Autodesk Inventor part; units mm, degrees
ref_plane "YZ Plane" through (0, 0, 0) normal (1, 0, 0) x (0, 1, 0)
ref_plane "XZ Plane" through (0, 0, 0) normal (0, 1, 0) x (-1, 0, 0)
ref_plane "XY Plane" through (0, 0, 0) normal (0, 0, 1) x (1, 0, 0)
sketch "草图1" plane through (0, 0, 0) normal (0, 0, 1) x (1, 0, 0)
  circle A0 centre (0, 0) radius 45
  dimension "d0" = 90
extrude "拉伸1" add sketch "草图1" along normal blind 7
sketch "草图2" plane through (0, 0, 7) normal (0, 0, 1) x (1, 0, 0)
  circle A0 centre (0, 0) radius 26
  circle A1 centre (0, 0) radius 21
  dimension "d3" = 52
  dimension "d4" = 42
extrude "拉伸2" add sketch "草图2" along normal blind 8
sketch "草图3" plane through (0, 0, 15) normal (0, 0, 1) x (1, 0, 0)
  circle A0 centre (0, 0) radius 26
  circle A1 centre (0, 0) radius 25
  dimension "d7" = 52
  dimension "d8" = 50
extrude "拉伸3" cut sketch "草图3" against normal blind 2
sketch "草图4" plane through (0, 0, 7) normal (0, 0, 1) x (1, 0, 0)
  circle A0 centre (0, 0) radius 13
  dimension "d11" = 26
extrude "拉伸4" cut sketch "草图4" against normal through all
sketch "草图5" plane through (0, 0, 0) normal (0, 0, -1) x (-1, 0, 0)
  circle A0 centre (0, -35.5) radius 2.5
  circle A1 centre (35.5, 0) radius 2.5
  circle A2 centre (-35.5, 0) radius 2.5
  circle A3 centre (0, 35.5) radius 2.5
  line L0 (0, 0) -> (-3.8614, 0)
  line L1 (0, 0) -> (0, -7.2667)
  dimension "d15" = 5
  dimension "d16" = 5
  dimension "d17" = 5
  dimension "d18" = 5
  dimension "d19" = 35.5
  dimension "d20" = 35.5
  dimension "d21" = 35.5
  dimension "d22" = 35.5
  dimension "d23" = 7.2667
  dimension "d24" = 3.8614
extrude "拉伸5" cut sketch "草图5" against normal through all
sketch "草图6" plane through (0, 0, 0) normal (0, 0, -1) x (-1, 0, 0)
  circle A0 centre (0, 0) radius 22.5
  dimension "d27" = 45
extrude "拉伸6" cut sketch "草图6" against normal blind 1
fillet "圆角1" radius 0.5 2 edges at (22.5, 0, 0) (22.5, 0, 1)
equation "\"d12\" = d11"
properties part number "装填盘轴盖"
Geometry: final body of the model. Coordinates: model frame, mm. A direction names the side the tool comes from. Coordinates: 2 decimals unless noted, no trailing zeros. Write each loop counter-clockwise with the first axis right and the second up, starting at its lowest first coordinate (ties: lowest second). Pieces come first, ordered by that corner, then holes. Notation, with made-up numbers: M 17,-20 L 54,-20 A14 ccw 54,-14 Z; hole C -31.5,78.25 d4. An arc over 180 degrees is marked long. Answer as CSV lines item,"result". Start each with the question number.
Q1. Mould query, pull axis Y, two halves, no side actions, for faces 1 (the cylindrical face through (-10.316, -7.91, 4.042)), 2 (the cylindrical face through (20.765, 39.923, 3.451)), 3 (the flat face through (-5.7, 20.5, 15)). Classes: released by +Y, released by -Y, zero draft, split by the parting line, or undercut.
Q2. Cut plane C-C on z = 5. Return the cut outline in (x, y).
Q3. Reachability of faces 4 (the flat face through (-9.5, -9.5, 1)), 5 (the flat face through (9, 10, 7)), 6 (the flat face through (-21, 11, 0)) from +Z, -Z, +X, -X, +Y, -Y: full face, straight path, thin tool, end or side. Return the list, or none.
Q4. Line query: line 1 (Y direction, x = 0, z = 2.6); line 2 (Z direction, x = -27.5, y = -23); line 3 (Y direction, x = 35.5, z = 3.25). Output: solid intervals per line, ascending. Write a range as from..to.
Q5. Cut plane B-B on x = 0. Count the separate pieces of the cut face and the enclosed holes in it, then the cut area to 3 significant figures.
Q6. Pin query (flat end, axial travel): P1, Ø15.5, axis at x = 7.5, y = 2.5, coming from the +Z side; P2, Ø5, axis at y = 22.5, z = 8.5, coming from the +X side; P3, Ø4, axis at y = -2.5, z = 11.5, coming from the +X side; P4, Ø1.5, axis at x = 34.5, y = 18, coming from the -Z side. Return the tip coordinate at first contact, or that it passes through.
Q7. Cut plane A-A on x = -35.5. Return the cut outline in (y, z), then the cut area to 3 significant figures.
Findings below:
1,face 1,"undercut"
1,face 2,"split by the parting line"
1,face 3,"zero draft"
2,outline,"C 0,0 d90; hole C -35.5,0 d5; hole C 0,0 d26; hole C 0,-35.5 d5; hole C 0,35.5 d5; hole C 35.5,0 d5"
3,face 4,"-Z"
3,face 5,"+Z"
3,face 6,"-Z, +X, -X, +Y, -Y"
4,line 1,"y = -45..-38, -33..-13, 13..33, 38..45"
4,line 2,"z = 0..7"
4,line 3,"y = -27.65..-2.5, 2.5..27.65"
5,separate pieces,"4"
5,enclosed holes,"0"
5,area,"435 mm2"
6,P1,"stops at z = 7"
6,P2,"stops at x = 40.06"
6,P3,"stops at x = 26"
6,P4,"stops at z = 0"
7,outline,"M -27.65,0 L -2.5,0 L -2.5,7 L -27.65,7 Z; M 2.5,0 L 27.65,0 L 27.65,7 L 2.5,7 Z"
7,area,"352 mm2"
